from build123d import *

# Parameters (mm, degrees)
BASE_FLANGE1_DEPTH   = 2
EDGE_FLANGE1_START   = -23
EDGE_FLANGE1_DEPTH   = 46
EDGE_FLANGE1_START_2 = -23.714787909
EDGE_FLANGE1_2_DEPTH = 0.714787909
EDGE_FLANGE1_START_3 = 23
EDGE_FLANGE1_3_DEPTH = 0.714787909
EDGE_FLANGE1_4_DEPTH = 46
CUT_EXTRUDE1_DEPTH   = 10
FILLET1_R            = 4
FILLET2_R            = 6
SKETCH9_R            = 3
CUT_EXTRUDE2_DEPTH   = 10
SKETCH10_R           = 3
BOSS_EXTRUDE1_DEPTH  = 2
SCALE1_SCALE         = 0.7761


# Read off the part's stored shape, not the designer's step: Edge-Flange1
# Sheet-metal steps are written as plain solids
with BuildPart() as part:
    # Sketch1 → Base-Flange1 (new body)
    with BuildSketch(Plane(origin=(0, 0, 0), x_dir=(1, 0, 0), z_dir=(0, 1, 0))):
        with BuildLine():
            Line((-16.949747468, 6.379735664), (-9, -1.570011804))
            Line((-9, -1.570011804), (9, -1.570011804))
            Line((9, -1.570011804), (16.949747468, 6.379735664))
            ThreePointArc((16.949747468, 6.379735664), (19.22071091, 7.897144924), (21.899494937, 8.429988196))
            Line((21.899494937, 8.429988196), (24, 8.429988196))
            ThreePointArc((24, 8.429988196), (27.535533906, 6.965522102), (29, 3.429988196))
            Line((29, 3.429988196), (29, -1.361639596))
            ThreePointArc((29, -1.361639596), (28.339066725, -3.564054954), (26.574683296, -5.038645514))
            Line((26.574683296, -5.038645514), (23, -6.569508994))
            Line((23, -6.569508994), (23, -10))
            Line((23, -10), (-23, -10))
            Line((-23, -10), (-23, -6.569508994))
            Line((-23, -6.569508994), (-26.574683296, -5.038645514))
            ThreePointArc((-26.574683296, -5.038645514), (-28.339066725, -3.564054954), (-29, -1.361639596))
            Line((-29, -1.361639596), (-29, 3.429988196))
            ThreePointArc((-29, 3.429988196), (-27.535533906, 6.965522102), (-24, 8.429988196))
            Line((-24, 8.429988196), (-21.899494937, 8.429988196))
            ThreePointArc((-21.899494937, 8.429988196), (-19.22071091, 7.897144924), (-16.949747468, 6.379735664))
        make_face()
    extrude(amount=-BASE_FLANGE1_DEPTH)

    # Edge-Flange1 outline → Edge-Flange1 (cut)
    with BuildSketch(Plane.YZ.offset(EDGE_FLANGE1_START)):
        with BuildLine():
            ThreePointArc((-2, 9.899002398), (-0.556604688, 8.917667209), (0, 7.2634))
            Line((0, 7.2634), (0, 10))
            Line((0, 10), (-2, 10))
            Line((-2, 10), (-2, 9.899002398))
        make_face()
    extrude(amount=EDGE_FLANGE1_DEPTH, mode=Mode.SUBTRACT)

    # Edge-Flange1 2 outline → Edge-Flange1 2 (cut)
    with BuildSketch(Plane.YZ.offset(EDGE_FLANGE1_START_2)):
        with BuildLine():
            Line((-2, 6.2634), (0, 6.2634))
            Line((0, 6.2634), (0, 7.2634))
            ThreePointArc((0, 7.2634), (-0.556604688, 8.917667209), (-2, 9.899002398))
            Line((-2, 9.899002398), (-2, 6.2634))
        make_face()
    extrude(amount=EDGE_FLANGE1_2_DEPTH, mode=Mode.SUBTRACT)

    # Edge-Flange1 3 outline → Edge-Flange1 3 (cut)
    with BuildSketch(Plane.YZ.offset(EDGE_FLANGE1_START_3)):
        with BuildLine():
            Line((-2, 6.2634), (0, 6.2634))
            Line((0, 6.2634), (0, 7.2634))
            ThreePointArc((0, 7.2634), (-0.556604688, 8.917667209), (-2, 9.899002398))
            Line((-2, 9.899002398), (-2, 6.2634))
        make_face()
    extrude(amount=EDGE_FLANGE1_3_DEPTH, mode=Mode.SUBTRACT)

    # Edge-Flange1 4 outline → Edge-Flange1 4 (add)
    with BuildSketch(Plane.YZ.offset(EDGE_FLANGE1_START)):
        with BuildLine():
            ThreePointArc((-2.7366, 8), (-2.215745145, 7.784254855), (-2, 7.2634))
            Line((-2, 7.2634), (-2, 9.899002398))
            ThreePointArc((-2, 9.899002398), (-2.364854094, 9.974633029), (-2.7366, 10))
            Line((-2.7366, 10), (-15, 10))
            Line((-15, 10), (-15, 8))
            Line((-15, 8), (-2.7366, 8))
        make_face()
    extrude(amount=EDGE_FLANGE1_4_DEPTH)

    # Sketch8 → Cut-Extrude1 (cut)
    with BuildSketch(Plane.XY.offset(10)):
        Polygon((-16, -10), (-23, -3), (-23, -15), (-5, -15), (-10, -10), align=None)
        Polygon((10, -10), (5, -15), (23, -15), (23, -3), (16, -10), align=None)
    extrude(amount=-CUT_EXTRUDE1_DEPTH, mode=Mode.SUBTRACT)

    # Fillet1
    fillet1_edges = [part.edges().sort_by_distance(p)[0] for p in [
        (-23, -3, 9),
        (-16, -10, 9),
        (-10, -10, 9),
        (10, -10, 9),
        (16, -10, 9),
        (23, -3, 9),
    ]]
    fillet(fillet1_edges, radius=FILLET1_R)

    # Fillet2
    fillet2_edges = [part.edges().sort_by_distance(p)[0] for p in [
        (-5, -15, 9),
        (5, -15, 9),
        (9, -1, 1.570011804),
        (-9, -1, 1.570011804),
    ]]
    fillet(fillet2_edges, radius=FILLET2_R)

    # Sketch9 → Cut-Extrude2 (cut)
    with BuildSketch(Plane.XY.offset(10)):
        with Locations((0, -9)):
            Circle(SKETCH9_R)
    extrude(amount=-CUT_EXTRUDE2_DEPTH, mode=Mode.SUBTRACT)

    # Sketch10 → Boss-Extrude1 (add)
    with BuildSketch(Plane(origin=(0, 0, 8), x_dir=(-1, 0, 0), z_dir=(0, 0, -1))):
        Polygon((5.42709253, -9), (2.713546265, -4.3), (-2.713546265, -4.3), (-5.42709253, -9), (-2.713546265, -13.7), (2.713546265, -13.7), align=None)
        with Locations(Location((0, -9, 0), (0, 0, 180))):
            Circle(SKETCH10_R, mode=Mode.SUBTRACT)
    extrude(amount=BOSS_EXTRUDE1_DEPTH)


with BuildPart() as part_1:
    # Scale1: scaled about (0, -3.290648573, 4.477741927)
    add(part.part.scale(SCALE1_SCALE).moved(Location((0, -0.736776215, 1.002566417))))


solid = part_1.part
Geometry check sheet. Reference: the model listing, model coordinates, mm. A direction names the side the tool comes from. Give positions to 0.01 mm unless a question says otherwise; leave off trailing zeros. Order: outer loops, then holes, each group sorted by start corner. A loop starts at its lowest first (then second) coordinate and runs counter-clockwise, first axis right, second up. Notation, with made-up numbers: (-31, 20) - (-18, 20) arc R20 cw to (-18, 53) - close; hole circle Ø9 at (25.5, -5). An arc over 180 degrees is marked (long way). Use one line per item in the form item = value.
1) Depth check by flat-ended pin: pin 1 Ø2 at (x, y) = (-13.5, -2.5) entering from -Z; pin 2 Ø4 at (y, z) = (-6, -3) entering from -X; pin 3 Ø1.2 at (x, z) = (1, 6.5) entering from -Y; pin 4 Ø0.5 at (y, z) = (-1.5, 6.5) entering from +X. Enter the tip coordinate at first touch or a pass-through.
Working result:
pin_1 = -4.92
pin_2 = through
pin_3 = -11.37
pin_4 = 17.85
2) Sectioned sample at A-A (x = 0). Record the boundary of the cut face in (y, z), and give its area (3 significant figures).
Working result:
outline = (-12.38, 7.21) - (-11.37, 7.21) - (-11.37, 5.66) - (-10.05, 5.66) - (-10.05, 8.76) - (-12.38, 8.76) - close; (-5.39, 5.66) - (-4.07, 5.66) - (-4.07, 7.21) - (-2.86, 7.21) arc R0.57 cw to (-2.29, 6.64) - (-2.29, 2.22) - (-0.74, 2.22) - (-0.74, 6.64) arc R2.12 ccw to (-2.86, 8.76) - (-5.39, 8.76) - close
area = 21.8 mm^2
3) Access from +Z, -Z, +X, -X, +Y, -Y to the whole of each face (thin tool, end or side, straight path). Record for faces 5 (the face through (-0.2, -3.5, 7.211)), 6 (the face through (0, -4, 8.764)), 7 (the face through (-6.862, -1.524, 1.857)), 8 (the face through (-3.144, -9.571, 6.446)), 9 (the face through (-17.85, -1, 7)).
Working result:
face_5 = -Z
face_6 = +Z, +X, -X, +Y, -Y
face_7 = -Z, +Y, -Y
face_8 = -Z, -X, -Y
face_9 = +Z, -X, +Y, -Y
4) Sectioned sample at D-D (x = 16.5). Record the boundary of the cut face in (y, z), and give its area (3 significant figures).
Working result:
outline = (-4.42, 7.21) - (-2.86, 7.21) arc R0.57 cw to (-2.29, 6.64) - (-2.29, -5.52) - (-0.74, -5.52) - (-0.74, 6.64) arc R2.12 ccw to (-2.86, 8.76) - (-4.42, 8.76) - close
area = 24.6 mm^2
5) Draft check along Y on faces 1 (the face through (0, -4.074, 6)), 2 (the face through (0, -0.737, 3)), 3 (the face through (18, -2, -5.54)), 4 (the face through (6.06, -10.2, 8)). Enter one of: released by +Y, released by -Y, zero draft, split by the parting line, or undercut.
Working result:
face_1 = undercut
face_2 = released by +Y
face_3 = zero draft
face_4 = released by -Y
6) Sectioned sample at B-B (z = 1.25). Record the boundary of the cut face in (x, y), and give its area (3 significant figures).
Working result:
outline = (-22.51, -2.29) - (-7.9, -2.29) - (-7.9, -0.74) - (-22.51, -0.74) - close; (7.9, -2.29) - (22.51, -2.29) - (22.51, -0.74) - (7.9, -0.74) - close
area = 45.3 mm^2
7) Sectioned sample at C-C (z = 8). Record the boundary of the cut face in (x, y), and give its area (3 significant figures).
Working result:
outline = (-17.85, -1.78) arc R3.1 ccw to (-16.94, -3.97) - (-13.33, -7.59) arc R3.1 ccw to (-11.13, -8.5) - (-9.05, -8.5) arc R3.1 cw to (-6.85, -9.41) - (-5.24, -11.01) arc R4.66 ccw to (-1.95, -12.38) - (1.95, -12.38) arc R4.66 ccw to (5.24, -11.01) - (6.85, -9.41) arc R3.1 cw to (9.05, -8.5) - (11.13, -8.5) arc R3.1 ccw to (13.33, -7.59) - (16.94, -3.97) arc R3.1 ccw to (17.85, -1.78) - (17.85, -1.23) - (-17.85, -1.23) - close; hole circle Ø4.66 at (0, -7.72)
area = 257 mm^2
8) Material ranges on probe 1 along Y at (x, z) = (0, 6.65); probe 2 along Z at (x, y) = (-13, -7.5); probe 3 along Y at (x, z) = (-19.5, -2.75), recorded low to high. Write a range as from..to.
Working result:
probe_1 = -11.37..-10.05, -5.39..-4.07, -2.29..-0.74
probe_2 = 7.21..8.76
probe_3 = -2.29..-0.74
